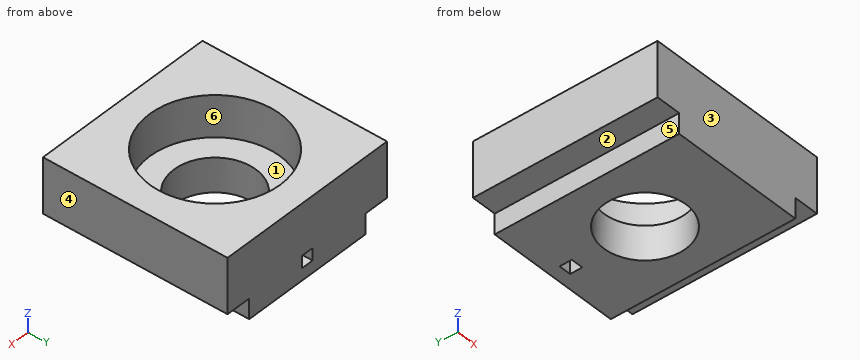
```python
from build123d import *

# Parameters (mm, degrees)
PAD_DEPTH       = 11.4
SKETCH002_W     = 1.5
SKETCH002_H     = 1.5
POCKET_DEPTH    = 3
SKETCH003_W     = 1.5
SKETCH003_H     = 1.5
POCKET001_DEPTH = 3


with BuildPart() as part:
    # Sketch → Pad (new body, symmetric)
    with BuildSketch(Plane.XZ):
        Polygon((-11.4, 9.3), (11.4, 9.3), (11.4, 2.5), (8.3, 2.5), (8.3, 0), (-8.3, 0), (-8.3, 2.5), (-11.4, 2.5), align=None)
    extrude(amount=PAD_DEPTH, both=True)

    # Sketch001 → Groove (revolve, cut)
    with BuildSketch(Plane.XZ):
        Polygon((0, 9.3), (8.05, 9.3), (8.05, 4.2), (5.05, 4.2), (5.05, 0), (0, 0), align=None)
    revolve(axis=Axis((0, 0, 0), (0, 0, 1)), mode=Mode.SUBTRACT)

    # Sketch002 → Pocket (cut)
    with BuildSketch(Plane(origin=(0, 0, 0), x_dir=(-1, 0, 0), z_dir=(0, 0, -1))):
        with Locations((0, 9.15)):
            Rectangle(SKETCH002_W, SKETCH002_H)
    extrude(amount=-POCKET_DEPTH, mode=Mode.SUBTRACT)

    # Sketch003 → Pocket001 (cut)
    with BuildSketch(Plane(origin=(0, 11.4, 0), x_dir=(-1, 0, 0), z_dir=(0, 1, 0))):
        with Locations((0, 2.25)):
            Rectangle(SKETCH003_W, SKETCH003_H)
    extrude(amount=-POCKET001_DEPTH, mode=Mode.SUBTRACT)


solid = part.part
```
Work out the finished part from the listing and answer in its coordinate system (mm). Face numbers are marked on the shaded views. A direction names the side the tool comes from. Give positions to 0.01 mm unless a question says otherwise; leave off trailing zeros. Order: outer loops, then holes, each group sorted by start corner. A loop starts at its lowest first (then second) coordinate and runs counter-clockwise, first axis right, second up. Notation, with made-up numbers: (-35.5, -23) - (-7.5, -23) arc R13 cw to (-7.5, -16) - close; hole circle Ø10 at (-31.5, -25). An arc over 180 degrees is marked (long way). One line per item, written item: value. Start each with the question number.
1. Section B-B, the plane z = 0.5 is taken. Write down the section's boundary in (x, y), then the cut area to 3 significant figures.
2. Section A-A, the plane x = 0 is taken. Write down the section's boundary in (y, z).
3. For a pull along X with two mould halves and no side action, classify the marked faces 4, 5 and 6 as released by +X, released by -X, zero draft, split by the parting line, or undercut.
4. Which of the six approach directions +Z, -Z, +X, -X, +Y, -Y give full straight-line access (tool end or side, diameter ignored) to the marked faces 1, 2 and 3?
5. Consider line 1 (Y direction, x = 0, z = 5.85); line 2 (Y direction, x = -2.5, z = 7.25); line 3 (X direction, y = 1.25, z = 2.75). Determine where each line is inside the solid, lowest interval first.
6. Section D-D, the plane x = -2.5 is taken. Write down the section's boundary in (y, z), then the cut area to 3 significant figures.
7. Each of these flat-tipped pins is pushed along its axis until it touches: pin 1 Ø2.5 at (y, z) = (9.5, 1) entering from -X; pin 2 Ø1.5 at (x, y) = (-10, 1) entering from -Z; pin 3 Ø8 at (x, y) = (0, -1.5) entering from +Z. Where does it stop, or does it pass through?
8. Section C-C, the plane y = 0 is taken. Write down the section's boundary in (x, z), then the cut area to 3 significant figures.
Filled sheet:
1. outline: (-8.3, -11.4) - (8.3, -11.4) - (8.3, 11.4) - (-8.3, 11.4) - close; hole circle Ø10.1 at (0, 0); hole (-0.75, 8.4) - (0.75, 8.4) - (0.75, 9.9) - (-0.75, 9.9) - close
1. area: 296 mm²
2. outline: (-11.4, 0) - (-5.05, 0) - (-5.05, 4.2) - (-8.05, 4.2) - (-8.05, 9.3) - (-11.4, 9.3) - close; (5.05, 0) - (8.4, 0) - (8.4, 3) - (11.4, 3) - (11.4, 9.3) - (8.05, 9.3) - (8.05, 4.2) - (5.05, 4.2) - close; (9.9, 0) - (11.4, 0) - (11.4, 1.5) - (9.9, 1.5) - close
3. face 4: released by +X
3. face 5: released by -X
3. face 6: undercut
4. face 1: +Z
4. face 2: -Z, -X, +Y, -Y
4. face 3: +Z, -Z, +X, -X, -Y
5. line 1: -11.4 to -8.05, 8.05 to 11.4
5. line 2: -11.4 to -7.65, 7.65 to 11.4
5. line 3: -11.4 to -4.89, 4.89 to 11.4
6. outline: (-11.4, 0) - (-4.39, 0) - (-4.39, 4.2) - (-7.65, 4.2) - (-7.65, 9.3) - (-11.4, 9.3) - close; (4.39, 0) - (11.4, 0) - (11.4, 9.3) - (7.65, 9.3) - (7.65, 4.2) - (4.39, 4.2) - close
6. area: 97.1 mm²
7. pin 1: x = -8.3
7. pin 2: z = 2.5
7. pin 3: z = 4.2
8. outline: (-11.4, 2.5) - (-8.3, 2.5) - (-8.3, 0) - (-5.05, 0) - (-5.05, 4.2) - (-8.05, 4.2) - (-8.05, 9.3) - (-11.4, 9.3) - close; (5.05, 0) - (8.3, 0) - (8.3, 2.5) - (11.4, 2.5) - (11.4, 9.3) - (8.05, 9.3) - (8.05, 4.2) - (5.05, 4.2) - close
8. area: 72.0 mm²
